Source: three-view drawing plus pictorial views. Frame: mm from the lowest corner of the part. A direction names the side the tool comes from. Give positions to 0.01 mm unless a question says otherwise; leave off trailing zeros. Order: outer loops, then holes, each group sorted by start corner. A loop starts at its lowest first (then second) coordinate and runs counter-clockwise, first axis right, second up. Notation, with made-up numbers: (47.5, 29.25) -> (80.5, 29.25) arc R17 ccw to (80.5, 51.25) -> close; hole circle Ø2 at (40.5, 87). An arc over 180 degrees is marked (long way). Answer in a Markdown table with one row per item. Add a question column.
Q1. Cut plane B-B on y = 5.5. Return the cut outline in (x, z) (3 decimals).
Q2. Cut plane D-D on x = 58.5. Return the cut outline in (y, z) (3 decimals).
Q3. Line query: line 1 along X through (y, z) = (10, 60); line 2 along Y through (x, z) = (38.1, 79.5) (3 decimals); line 3 along Y through (x, z) = (37.5, 14.5). Output: solid intervals per line, ascending. Write a range as from..to.
Q4. Contact query for flat-ended pins moving along their axis: P1, Ø2, axis at x = 68.5, y = 7.5, coming from the -Z side (3 decimals); P2, Ø4, axis at x = 23, z = 81, coming from the +Y side; P3, Ø5, axis at y = 13.5, z = 4, coming from the -X side; P4, Ø9.5, axis at x = 70, y = 10, coming from the +Z side (3 decimals). Output: stop coordinate, or through.
Q5. Set-up query: the marked faces 1, 2 and 3. Return all of +Z, -Z, +X, -X, +Y, -Y with unobstructed straight access to the full face (end or side cutting, diameter ignored); none if empty.
Q6. Cut plane C-C on z = 48.5. Return the cut outline in (x, y) (3 decimals).
Q7. Cut plane A-A on x = 38.1. Return the cut outline in (y, z) (3 decimals), and give its area (3 significant figures).
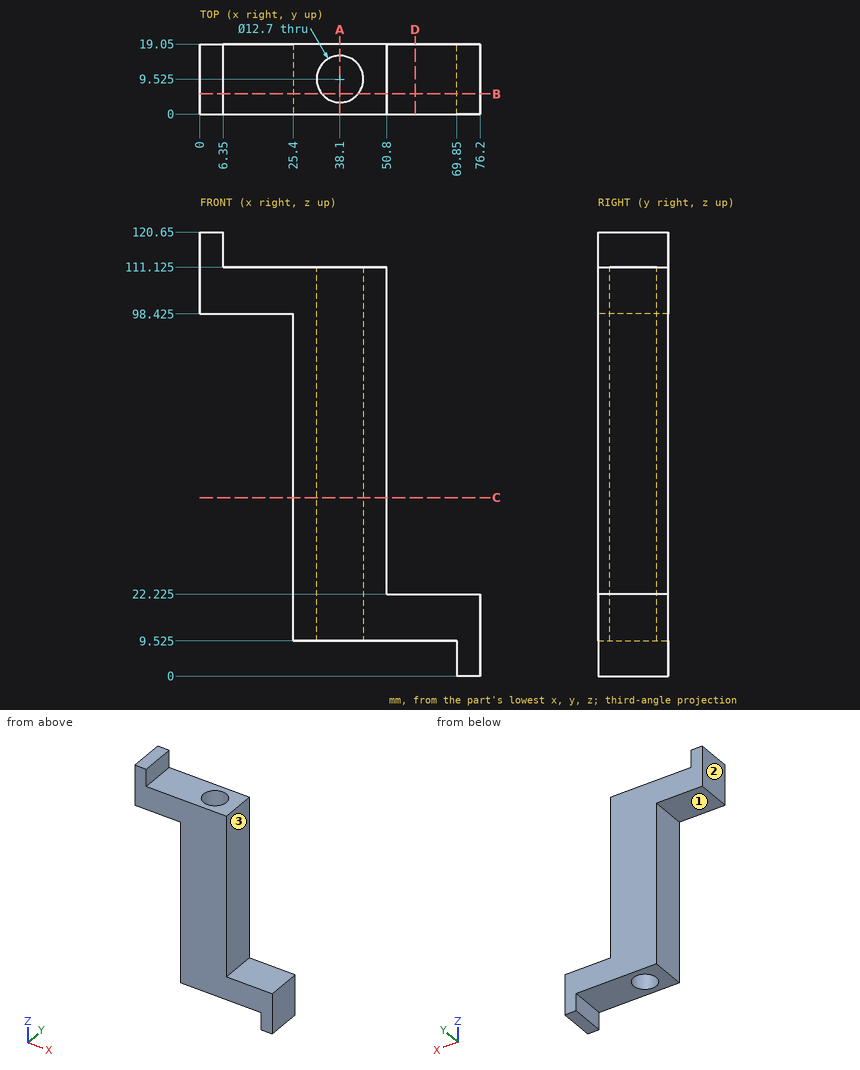
Completed:
| question | item | result |
|---|---|---|
| 1 | outline | (0, 98.425) -> (25.4, 98.425) -> (25.4, 9.525) -> (33.189, 9.525) -> (33.189, 111.125) -> (6.35, 111.125) -> (6.35, 120.65) -> (0, 120.65) -> close; (43.011, 9.525) -> (69.85, 9.525) -> (69.85, 0) -> (76.2, 0) -> (76.2, 22.225) -> (50.8, 22.225) -> (50.8, 111.125) -> (43.011, 111.125) -> close |
| 2 | outline | (0, 9.525) -> (19.05, 9.525) -> (19.05, 22.225) -> (0, 22.225) -> close |
| 3 | line 1 | x = 25.4..31.77, 44.43..50.8 |
| 3 | line 2 | y = 0..3.175, 15.875..19.05 |
| 3 | line 3 | y = 0..3.2, 15.85..19.05 |
| 4 | P1 | stops at z = 9.525 |
| 4 | P2 | passes through |
| 4 | P3 | stops at x = 69.85 |
| 4 | P4 | stops at z = 22.225 |
| 5 | face 1 | -Z, -X, +Y, -Y |
| 5 | face 2 | +Z, -Z, -X, +Y, -Y |
| 5 | face 3 | +Z, +X, +Y, -Y |
| 6 | outline | (25.4, 0) -> (50.8, 0) -> (50.8, 19.05) -> (25.4, 19.05) -> close; hole circle Ø12.7 at (38.1, 9.525) |
| 7 | outline | (0, 9.525) -> (3.175, 9.525) -> (3.175, 111.125) -> (0, 111.125) -> close; (15.875, 9.525) -> (19.05, 9.525) -> (19.05, 111.125) -> (15.875, 111.125) -> close |
| 7 | area | 645 mm² |
